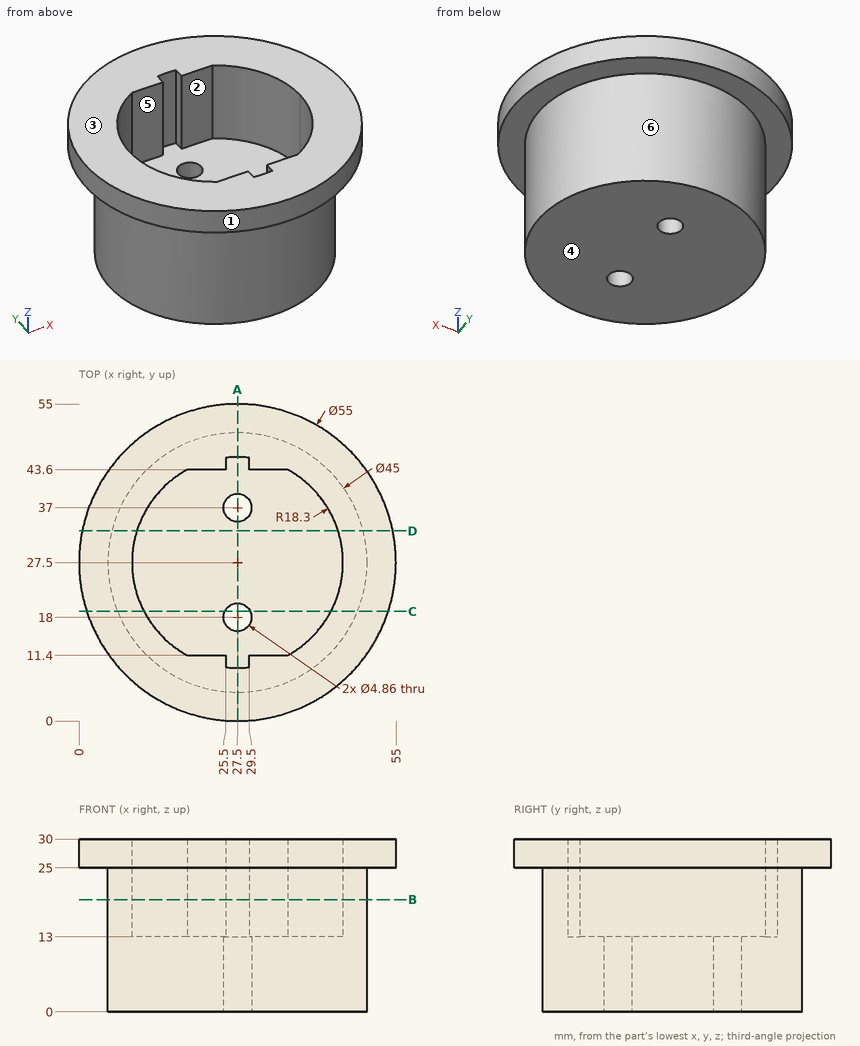
Check sheet for the drawn part. Datum: minimum x, y, z corner. Units: mm. A direction names the side the tool comes from. Give positions to 0.01 mm unless a question says otherwise; leave off trailing zeros. Loops run counter-clockwise (first coordinate to the right, second up) from the corner with the lowest first, then second, coordinate; pieces in that order, holes last. Notation, with made-up numbers: (-26, -23) - (19, -23) arc R15 cw to (19, -11) - close; hole circle Ø2 at (81.25, 78.25). An arc over 180 degrees is marked (long way). Write each question's results on one line, items separated by ' | '.
1) Tool access check on the marked faces 4, 5 and 6. Record the directions out of +Z, -Z, +X, -X, +Y, -Y that give a thin tool (end or side, any length) a straight path to the whole face; none if there is none.
Solution:
face 4: -Z, +X, -X, +Y, -Y | face 5: +Z | face 6: -Z
2) Sectioned sample at D-D on y = 33. Record the boundary of the cut face in (x, z), plus the area to 3 significant figures.
Solution:
outline: (0.56, 25) - (5.68, 25) - (5.68, 0) - (49.32, 0) - (49.32, 25) - (54.44, 25) - (54.44, 30) - (44.95, 30) - (44.95, 13) - (10.05, 13) - (10.05, 30) - (0.56, 30) - close | area: 767 mm2
3) Mould release check, pull along Y, two halves, no side actions. Record for the marked faces 1, 2 and 3: pulls with the +Y half, pulls with the -Y half, needs draft (parallel to the pull), parting line crosses it, or undercut.
Solution:
face 1: parting line crosses it | face 2: undercut | face 3: needs draft
4) Sectioned sample at A-A on x = 27.5. Record the boundary of the cut face in (y, z), plus the area to 3 significant figures.
Solution:
outline: (0, 25) - (5, 25) - (5, 0) - (15.57, 0) - (15.57, 13) - (9.2, 13) - (9.2, 30) - (0, 30) - close; (20.43, 0) - (34.57, 0) - (34.57, 13) - (20.43, 13) - close; (39.43, 0) - (50, 0) - (50, 25) - (55, 25) - (55, 30) - (45.8, 30) - (45.8, 13) - (39.43, 13) - close | area: 651 mm2
5) Sectioned sample at C-C on y = 19. Record the boundary of the cut face in (x, z), plus the area to 3 significant figures.
Solution:
outline: (1.35, 25) - (6.67, 25) - (6.67, 0) - (25.29, 0) - (25.29, 13) - (11.29, 13) - (11.29, 30) - (1.35, 30) - close; (29.71, 0) - (48.33, 0) - (48.33, 25) - (53.65, 25) - (53.65, 30) - (43.71, 30) - (43.71, 13) - (29.71, 13) - close | area: 695 mm2
6) Sectioned sample at B-B on z = 19.5. Record the boundary of the cut face in (x, y).
Solution:
outline: circle Ø45 at (27.5, 27.5); hole (18.8, 11.4) - (25.5, 11.4) - (25.5, 9.31) arc R18.3 ccw to (29.5, 9.31) - (29.5, 11.4) - (36.2, 11.4) arc R18.3 ccw to (36.2, 43.6) - (29.5, 43.6) - (29.5, 45.69) arc R18.3 ccw to (25.5, 45.69) - (25.5, 43.6) - (18.8, 43.6) arc R18.3 ccw to start
7) Material ranges on L1, parallel to Y at x = 27.5, z = 8.5; L2, parallel to Y at x = 16, z = 21.75; L3, parallel to X at y = 11, z = 27.5, recorded low to high. Write a range as from..to.
Solution:
L1: 5..15.57, 20.43..34.57, 39.43..50 | L2: 8.16..13.26, 41.74..46.84 | L3: 5.5..25.5, 29.5..49.5
8) Depth check by flat-ended pin: P1, Ø7.5, axis at x = 22.5, z = 24.5, coming from the +Y side; P2, Ø8, axis at x = 28.5, z = 19.5, coming from the +Y side; P3, Ø6, axis at x = 22, z = 12.5, coming from the -Y side; P4, Ø16.5, axis at x = 33.5, y = 14.5, coming from the -Z side. Enter the tip coordinate at first touch or a pass-through.
Solution:
P1: y = 54.97 | P2: y = 50 | P3: y = 5.14 | P4: z = 0
